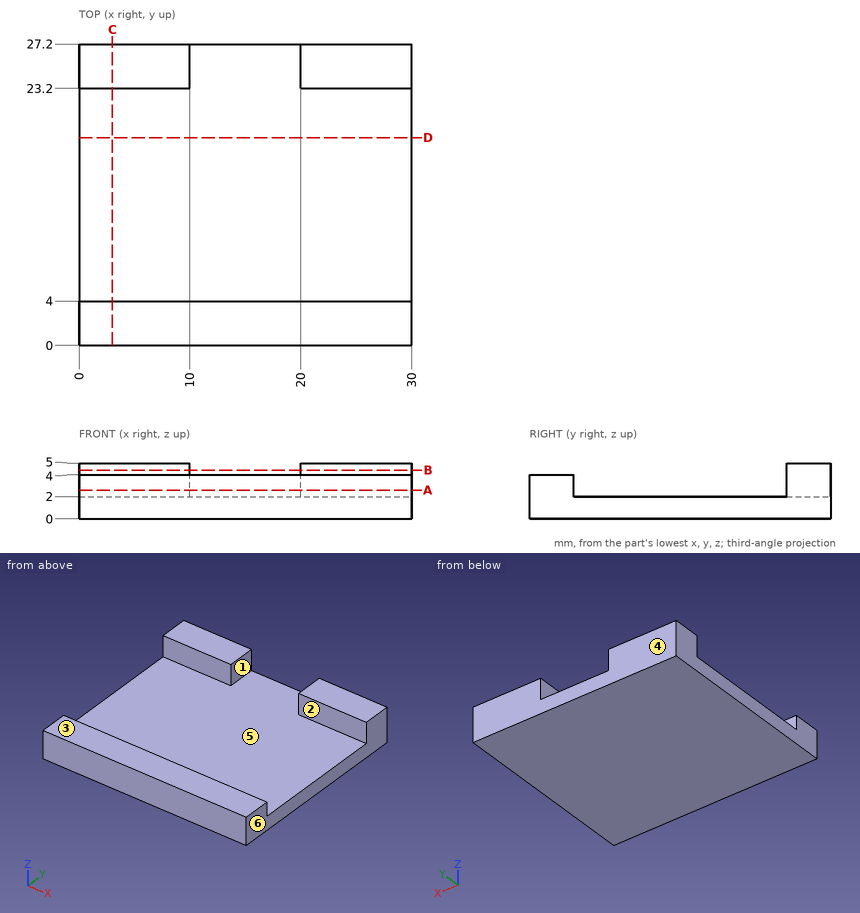
Here's the drawing with two shaded views (mm, measured from the low corner). I have some questions. A direction names the side the tool comes from. Round coordinates to 2 decimals unless told otherwise and drop trailing zeros. Write each loop counter-clockwise with the first axis right and the second up, starting at its lowest first coordinate (ties: lowest second). Pieces come first, ordered by that corner, then holes.
(1) For pin 1 (1.5 mm diameter, centred on y = 16.5, z = 3.5, fed in from -X); pin 2 (2 mm diameter, centred on x = 14, y = 1, fed in from +Z); pin 3 (1 mm diameter, centred on x = 14, y = 8.5, fed in from +Z); pin 4 (0.6 mm diameter, centred on x = 11.5, z = 3, fed in from +Y), each with a flat end and sliding along its axis, tell me the tip position at first contact or that it passes through.
Findings below:
pin 1: passes through
pin 2: stops at z = 4
pin 3: stops at z = 2
pin 4: stops at y = 4
(2) Suppose I cut it at A-A on z = 2.6. Write out the boundary of the cut face in (x, y).
Findings below:
outline: (0, 0) - (30, 0) - (30, 4) - (0, 4) - close; (0, 23.2) - (10, 23.2) - (10, 27.2) - (0, 27.2) - close; (20, 23.2) - (30, 23.2) - (30, 27.2) - (20, 27.2) - close
(3) Suppose I cut it at D-D on y = 18.75. Write out the boundary of the cut face in (x, z).
Findings below:
outline: (0, 0) - (30, 0) - (30, 2) - (0, 2) - close
(4) Thinking about a two-plate mould opening in Y: for the marked faces 4, 5 and 6, which applies, +Y half, -Y half, draft (parallel to the pull), parting line (faces both ways), or undercut?
Findings below:
face 4: +Y half
face 5: undercut
face 6: draft
(5) Suppose I cut it at C-C on x = 3. Write out the boundary of the cut face in (y, z), and give its area (3 significant figures).
Findings below:
outline: (0, 0) - (27.2, 0) - (27.2, 5) - (23.2, 5) - (23.2, 2) - (4, 2) - (4, 4) - (0, 4) - close
area: 74.4 mm2
(6) If I drill on probe 1 along Y at (x, z) = (26.25, 2.35); probe 2 along Z at (x, y) = (11.25, 14.5); probe 3 along Y at (x, z) = (6.5, 4.45), over which ranges is the centre line in solid material (lowest first)?
Findings below:
probe 1: y = 0 to 4, 23.2 to 27.2
probe 2: z = 0 to 2
probe 3: y = 23.2 to 27.2
(7) Which directions (+Z, -Z, +X, -X, +Y, -Y) give clear straight access to the entire face, cutting with the end or side of a thin tool? Please do the marked faces 1, 2 and 3.
Findings below:
face 1: +Z, +Y
face 2: +Z, +X, -X
face 3: +Z, +X, -X, -Y
(8) Suppose I cut it at B-B on z = 4.4. Write out the boundary of the cut face in (x, y).
Findings below:
outline: (0, 23.2) - (10, 23.2) - (10, 27.2) - (0, 27.2) - close; (20, 23.2) - (30, 23.2) - (30, 27.2) - (20, 27.2) - close
